Can you work these out from the model? Positions are in its coordinate system, mm. A direction names the side the tool comes from. Round coordinates to 2 decimals unless told otherwise and drop trailing zeros. Order: outer loops, then holes, each group sorted by start corner. A loop starts at its lowest first (then second) coordinate and runs counter-clockwise, first axis right, second up. Notation, with made-up numbers: M 2.5,-30.5 L 49.5,-30.5 A28 ccw 49.5,5.5 Z; hole C 24,-35 d5. An arc over 180 degrees is marked long. One line per question, with ' | ' between items.
Autodesk Inventor part; units mm, degrees
ref_plane "YZ Plane" through (0, 0, 0) normal (1, 0, 0) x (0, 1, 0)
ref_plane "XZ Plane" through (0, 0, 0) normal (0, 1, 0) x (-1, 0, 0)
ref_plane "XY Plane" through (0, 0, 0) normal (0, 0, 1) x (1, 0, 0)
sketch "Sketch1" plane through (0, 0, 0) normal (0, 0, 1) x (1, 0, 0)
  line L0 (-232, 103.6) -> (18, 103.6)
  line L1 (18, 103.6) -> (18, -146.4)
  line L2 (18, -146.4) -> (-232, -146.4)
  line L3 (-232, -146.4) -> (-232, 103.6)
  line L4 (0, -128.4) -> (0, 85.6)
  line L5 (0, -128.4) -> (-214, -128.4)
  line L6 (-214, -128.4) -> (0, -128.4)
  line L7 (18, 85.6) -> (18, 64.2)
  line L8 (18, 64.2) -> (0, 64.2)
  line L9 (0, 64.2) -> (0, 85.6)
  line L10 (18, 21.4) -> (0, 21.4)
  line L11 (0, 21.4) -> (0, 0)
  line L12 (0, 0) -> (18, 0)
  line L13 (0, -42.8) -> (18, -42.8)
  line L14 (18, -64.2) -> (0, -64.2)
  line L15 (18, -107) -> (0, -107)
  line L16 (-232, 103.6) -> (-232, 85.6)
  line L17 (0, 85.6) -> (0, 103.6)
  line L18 (-232, -107) -> (-214, -107)
  line L19 (-232, -64.2) -> (-214, -64.2)
  line L20 (-214, -42.8) -> (-232, -42.8)
  line L21 (-214, 0) -> (-232, 0)
  line L22 (-232, 21.4) -> (-214, 21.4)
  line L23 (-232, 64.2) -> (-214, 64.2)
  line L24 (-85.6, -128.4) -> (-85.6, -146.4)
  line L25 (-128.4, -128.4) -> (-128.4, -146.4)
  line L26 (-149.8, -146.4) -> (-149.8, -128.4)
  line L27 (-192.6, -146.4) -> (-192.6, -128.4)
  line L28 (-64.2, -146.4) -> (-64.2, -128.4)
  line L29 (-21.4, -146.4) -> (-21.4, -128.4)
  line L30 (-85.6, 103.6) -> (-85.6, 85.6)
  line L31 (-64.2, 85.6) -> (-64.2, 103.6)
  line L32 (-21.4, 85.6) -> (-21.4, 103.6)
  line L33 (-149.8, 85.6) -> (-149.8, 103.6)
  line L34 (-192.6, 85.6) -> (-192.6, 103.6)
  line L35 (-128.4, 103.6) -> (-128.4, 85.6)
  line L36 (0, 85.6) -> (-214, 85.6)
  line L37 (-214, 85.6) -> (-214, -128.4)
  line L38 (0, 85.6) -> (18, 85.6)
  line L39 (18, 85.6) -> (18, 103.6)
  line L40 (18, 103.6) -> (0, 103.6)
  line L41 (0, 103.6) -> (0, 85.6)
  line L42 (0, -128.4) -> (18, -128.4)
  line L43 (18, -128.4) -> (18, -146.4)
  line L44 (18, -146.4) -> (0, -146.4)
  line L45 (0, -146.4) -> (0, -128.4)
  line L46 (-214, -128.4) -> (-232, -128.4)
  line L47 (-232, -128.4) -> (-232, -146.4)
  line L48 (-232, -146.4) -> (-214, -146.4)
  line L49 (-214, -146.4) -> (-214, -128.4)
  line L50 (-214, 85.6) -> (-232, 85.6)
  line L51 (-232, 85.6) -> (-232, 103.6)
  line L52 (-232, 103.6) -> (-214, 103.6)
  line L53 (-214, 103.6) -> (-214, 85.6)
  point P0 (0, 0)
  point P1 (248.5081, 104.1116)
  point P2 (266.5081, 104.1116)
  point P3 (248.5081, 146.9116)
  point P4 (227.1081, 168.3116)
  point P5 (227.1081, 186.3116)
  point P6 (184.3081, 186.3116)
  point P7 (184.3081, 168.3116)
  point P8 (162.9081, 168.3116)
  point P9 (162.9081, 186.3116)
  point P10 (120.1081, 186.3116)
  point P11 (120.1081, 168.3116)
  point P12 (98.7081, 168.3116)
  point P13 (98.7081, 186.3116)
  point P14 (55.9081, 186.3116)
  point P15 (55.9081, 168.3116)
  point P16 (34.5081, 146.9116)
  point P17 (16.5081, 146.9116)
  point P18 (16.5081, 104.1116)
  point P19 (34.5081, 104.1116)
  point P20 (34.5081, 82.7116)
  point P21 (16.5081, 82.7116)
  point P22 (16.5081, 39.9116)
  point P23 (34.5081, 39.9116)
  point P24 (34.5081, 18.5116)
  point P25 (16.5081, 18.5116)
  point P26 (16.5081, -24.2884)
  point P27 (34.5081, -24.2884)
  point P28 (34.5081, -45.6884)
  point P29 (55.9081, -45.6884)
  point P30 (55.9081, -63.6884)
  point P31 (98.7081, -63.6884)
  point P32 (98.7081, -45.6884)
  point P33 (120.1081, -45.6884)
  point P34 (120.1081, -63.6884)
  point P35 (162.9081, -63.6884)
  point P36 (162.9081, -45.6884)
  point P37 (184.3081, -45.6884)
  point P38 (184.3081, -63.6884)
  point P39 (227.1081, -63.6884)
  point P40 (227.1081, -45.6884)
  point P41 (248.5081, -45.6884)
  point P42 (248.5081, -24.2884)
  point P43 (266.5081, -24.2884)
  point P44 (266.5081, 18.5116)
  point P45 (248.5081, 18.5116)
  point P46 (248.5081, 39.9116)
  point P47 (266.5081, 39.9116)
  point P48 (266.5081, 82.7116)
  point P49 (248.5081, 82.7116)
  dimension "d0" = 250
  dimension "d1" = 250
  dimension "d2" = 21.4
extrude "Plate1" add sketch "Sketch1" against normal blind 18 contours L0 L53 L50 L3 | L0 L34 L36 L53 | L0 L33 L36 L34 | L36 L4 L5 L37 | L23 L37 L22 L3 | L0 L30 L36 L35 | L21 L37 L20 L3 | L0 L32 L36 L31 | L19 L37 L18 L3 | L0 L17 L36 L32 | L18 L37 L46 L3 | L0 L1 L38 L17 | L46 L49 L2 L3 | L5 L27 L2 L49 | L8 L1 L10 L4 | L5 L26 L2 L27 | L12 L1 L13 L4 | L5 L24 L2 L25 | L14 L1 L15 L4 | L5 L29 L2 L28 | L5 L45 L2 L29 | L42 L1 L2 L45
sketch "Sketch2" plane through (0, 0, 0) normal (0, 0, 1) x (1, 0, 0)
  line L0 (-232, 0) -> (-232, -42.8)
  line L1 (-128.4, 85.6) -> (-149.8, 85.6)
  line L2 (-149.8, -128.4) -> (-128.4, -128.4)
  line L3 (-128.4, 85.6) -> (-128.4, -128.4)
  line L4 (-128.4, 85.6) -> (-128.4, -21.4)
  line L5 (-137.4, 53.5) -> (-119.4, 53.5)
  line L6 (-119.4, 53.5) -> (-119.4, 10.7)
  line L7 (-119.4, 10.7) -> (-137.4, 10.7)
  line L8 (-137.4, 10.7) -> (-137.4, 53.5)
  line L9 (-137.4, 53.5) -> (-119.4, 10.7) construction
  line L10 (-119.4, 53.5) -> (-137.4, 10.7) construction
  line L11 (-128.4, -128.4) -> (-128.4, -21.4)
  line L12 (-128.4, -21.4) -> (-128.4, -74.9)
  line L13 (-137.4, -96.3) -> (-119.4, -96.3)
  line L14 (-119.4, -96.3) -> (-119.4, -53.5)
  line L15 (-119.4, -53.5) -> (-137.4, -53.5)
  line L16 (-137.4, -53.5) -> (-137.4, -96.3)
  line L17 (-137.4, -96.3) -> (-119.4, -53.5) construction
  line L18 (-119.4, -96.3) -> (-137.4, -53.5) construction
  point P0 (0, 0)
  point P1 (-232, 103.6)
  point P2 (-128.4, 32.1)
  point P3 (-232, 103.6)
  dimension "d4" = 18
  dimension "d5" = 42.8
  dimension "d6" = 42.8
extrude "Cut1" cut sketch "Sketch2" against normal blind 18
sketch "Sketch3" plane through (0, 0, 0) normal (0, 0, 1) x (1, 0, 0)
  line L0 (-232, -128.4) -> (-214, -128.4)
  line L1 (-214, -128.4) -> (-214, -107)
  line L2 (-214, -128.4) -> (-214, -107)
  line L3 (-232, -107) -> (-214, -107)
  line L4 (-232, -107) -> (-232, -128.4)
  point P0 (0, 0)
extrude "Cut2" cut sketch "Sketch3" against normal blind 18
equation "\"d7\" = Thickness"
equation "\"d9\" = Thickness"
equation "\"d3\" = Thickness"
equation "\"BendRadius\" = Thickness"
equation "\"BendReliefWidth\" = Thickness"
equation "\"BendReliefDepth\" = 0.5 * Thickness"
equation "\"CornerReliefSize\" = 4 * Thickness"
equation "\"MinimumRemnant\" = 2 * Thickness"
equation "\"TransitionRadius\" = BendRadius"
equation "\"JacobiRadiusSize\" = BendRadius"
equation "\"GapSize\" = Thickness"
properties part number "1"
(1) If we section it at C-C on y = 82.5: Please give me the cut outline in (x, z), plus the area to 3 significant figures.
Final values:
outline: M -214,-18 L 0,-18 L 0,0 L -214,0 Z | area: 3,850 mm^2
(2) On a 3-axis mill with a long thin cutter (end or side, diameter ignored), from which of +Z, -Z, +X, -X, +Y, -Y can I reach the whole of each face in a straight line? I mean faces 1 (the flat face through (-119.4, -75, -9)), 2 (the flat face through (-75, -128.4, -9)), 3 (the flat face through (-214, 75, -9)). Say none if no direction works.
Final values:
face 1: +Z, -Z | face 2: +Z, -Z, -Y | face 3: +Z, -Z, -X
(3) Thinking about a two-plate mould opening in X: for faces 4 (the flat face through (0, 11, -9)), 5 (the flat face through (-149.8, 94, -9)), 6 (the flat face through (-107, 103.6, -9)), which applies, released by +X, released by -X, zero draft, split by the parting line, or undercut?
Final values:
face 4: released by +X | face 5: undercut | face 6: zero draft
(4) Please list where these lines run through material, in increasing order: probe 1 along Y at (x, z) = (5, -9.5); probe 2 along X at (y, z) = (43, -9); probe 3 along X at (y, z) = (-135, -2.25). Write a range as [from, to].
Final values:
probe 1: [-146.4, -128.4], [-107, -64.2], [-42.8, 0], [21.4, 64.2], [85.6, 103.6] | probe 2: [-232, -137.4], [-119.4, 18] | probe 3: [-232, -149.8], [-128.4, -85.6], [-64.2, 18]
(5) Will these pins go through, and if not, where does the flat tip stop? pin 1 Ø9 at (y, z) = (75, -8.5) entering from +X; pin 2 Ø2 at (x, z) = (-75, -15.5) entering from -Y; pin 3 Ø5.5 at (x, z) = (-138.5, -6.5) entering from +Y.
Final values:
pin 1: x = 0 | pin 2: y = -128.4 | pin 3: y = 85.6
(6) If we section it at A-A on y = 29.5: Please give me the cut outline in (x, z).
Final values:
outline: M -232,-18 L -137.4,-18 L -137.4,0 L -232,0 Z; M -119.4,-18 L 18,-18 L 18,0 L -119.4,0 Z
(7) If we section it at B-B on z = -13.75: State how many separate pieces and enclosed holes the cut face has, plus the area to 3 significant figures.
Final values:
separate pieces: 1 | enclosed holes: 2 | area: 56,300 mm^2
